Part model, mm, in its own coordinate system. A direction names the side the tool comes from. Round coordinates to 2 decimals unless told otherwise and drop trailing zeros. Loops run counter-clockwise (first coordinate to the right, second up) from the corner with the lowest first, then second, coordinate; pieces in that order, holes last.
1) Band-saw the part on D-D, the plane z = 3.75. Write the cut outline in (x, y).
2) Mould opens along X. For faces 1 (the flat face through (0, 2, -3)), 2 (the cylindrical face through (-13, 1, 0)), 3 (the cylindrical face through (-11, 1, 0)) say: +X half, -X half, draft (parallel to the pull), parting line (faces both ways), or undercut.
3) Band-saw the part on A-A, the plane x = -8.5. Write the cut outline in (y, z).
4) 3-axis set-ups, long thin cutter, end or side, ignore diameter. For faces 4 (the flat face through (0, 1, 4)), 5 (the flat face through (0, 1, 2)): which of +Z, -Z, +X, -X, +Y, -Y reach the whole face in a straight line?
5) Band-saw the part on C-C, the plane y = 0.4. Write the cut outline in (x, z).
6) Probe line 1 (Z direction, x = -1.25, y = 1.9); line 2 (X direction, y = 0.25, z = 0); line 3 (X direction, y = 0.4, z = -1.5). List the from-to ranges inside material, lowest first.
7) Band-saw the part on B-B, the plane z = 0. Write the cut outline in (x, y), then the cut area to 3 significant figures.
from build123d import *

# Parameters (mm, degrees)
BOSS_EXTRUDE1_DEPTH = 2


with BuildPart() as part:
    # Sketch1 → Boss-Extrude1 (new body)
    with BuildSketch(Plane(origin=(0, 0, 0), x_dir=(1, 0, 0), z_dir=(0, 1, 0))):
        with BuildLine():
            ThreePointArc((9, -4), (13, 0), (9, 4))
            Line((9, 4), (-9, 4))
            ThreePointArc((-9, 4), (-13, 0), (-9, -4))
            Line((-9, -4), (9, -4))
        make_face()
        with BuildLine():
            Line((-9, 2), (9, 2))
            ThreePointArc((9, 2), (11, 0), (9, -2))
            Line((9, -2), (-9, -2))
            ThreePointArc((-9, -2), (-11, 0), (-9, 2))
        make_face(mode=Mode.SUBTRACT)
    extrude(amount=BOSS_EXTRUDE1_DEPTH)


solid = part.part
Reported:
1. outline: (-10.39, 0) - (10.39, 0) - (10.39, 2) - (-10.39, 2) - close
2. face 1: draft
2. face 2: -X half
2. face 3: undercut
3. outline: (0, -4) - (2, -4) - (2, -2) - (0, -2) - close; (0, 2) - (2, 2) - (2, 4) - (0, 4) - close
4. face 4: +Z, +X, -X, +Y, -Y
4. face 5: +Y, -Y
5. outline: (-9, -4) - (9, -4) arc R4 ccw to (9, 4) - (-9, 4) arc R4 ccw to start; hole (-9, -2) - (9, -2) arc R2 ccw to (9, 2) - (-9, 2) arc R2 ccw to start
6. line 1: z = -4 to -2, 2 to 4
6. line 2: x = -13 to -11, 11 to 13
6. line 3: x = -12.71 to -10.32, 10.32 to 12.71
7. outline: (-13, 0) - (-11, 0) - (-11, 2) - (-13, 2) - close; (11, 0) - (13, 0) - (13, 2) - (11, 2) - close
7. area: 8.00 mm2
